Model file for the job. Use its own axes, mm. Face numbers are marked on the shaded views. Round coordinates to 2 decimals unless told otherwise and drop trailing zeros. Answer as a JSON object with one key per item and string values. Group by question number.
from build123d import *

# Parameters (mm, degrees)
ESQUISSE1_W        = 106.4
ESQUISSE1_H        = 74.1
BOSS_EXTRU_1_DEPTH = 27.7
CONG_2_R           = 13.85
CONG_3_R           = 1


with BuildPart() as part:
    # Esquisse1 → Boss.-Extru.1 (new body)
    with BuildSketch(Plane(origin=(0, 0, 0), x_dir=(1, 0, 0), z_dir=(0, 1, 0))):
        with Locations((53.2, 37.05)):
            Rectangle(ESQUISSE1_W, ESQUISSE1_H)
    extrude(amount=BOSS_EXTRU_1_DEPTH)

    # Congé2
    cong_2_edges = [part.edges().sort_by_distance(p)[0] for p in [
        (0, 0, -37.05),
        (0, 27.7, -37.05),
        (106.4, 27.7, -37.05),
        (106.4, 0, -37.05),
    ]]
    fillet(cong_2_edges, radius=CONG_2_R - 0.0001)  # a hair under: the kernel refuses the full size

    # Congé3
    cong_3_edges = [part.edges().sort_by_distance(p)[0] for p in [
        (53.2, 0, 0),
        (53.2, 27.7, 0),
        (102.343458209, 4.056541791, 0),
        (102.343458209, 23.643458209, 0),
        (4.056541791, 23.643458209, 0),
        (4.056541791, 4.056541791, 0),
        (53.2, 0, -74.1),
        (53.2, 27.7, -74.1),
        (102.343458209, 4.056541791, -74.1),
        (102.343458209, 23.643458209, -74.1),
        (4.056541791, 23.643458209, -74.1),
        (4.056541791, 4.056541791, -74.1),
    ]]
    fillet(cong_3_edges, radius=CONG_3_R)


solid = part.part
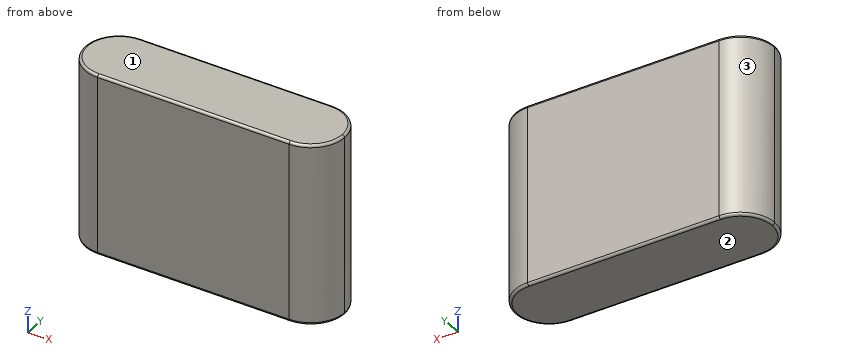
(1) Drill centre lines: line 1 (X direction, y = 24, z = -40.5); line 2 (Y direction, x = 12.5, z = -61); line 3 (X direction, y = 4.5, z = -60). Where is each one in solid material? Low to high. Write a range as from..to.
(2) Pull direction Z, two halves, no side cores. Call the marked faces 1, 2 and 3: pulls with the +Z half, pulls with the -Z half, needs draft (parallel to the pull), parting line crosses it, or undercut.
(3) Flat gauge pin, fed straight in: pin 1 (8 mm diameter, centred on y = 9.5, z = -51.5, fed in from +X). Where does the tip first touch, or does it go through?
Answer:
{
 "1": {"line 1": "4.43..101.97", "line 2": "0.07..27.63", "line 3": "3.63..102.77"},
 "2": {"face 1": "pulls with the +Z half", "face 2": "pulls with the -Z half", "face 3": "needs draft"},
 "3": {"pin 1": "x = 106.4"}
}
